The listing builds one solid part. Answer for the finished solid, in the listing's coordinates (mm). Give positions to 0.01 mm unless a question says otherwise; leave off trailing zeros. Loops run counter-clockwise (first coordinate to the right, second up) from the corner with the lowest first, then second, coordinate; pieces in that order, holes last.
Item 1: Each of these flat-tipped pins is pushed along its axis until it touches: pin 1 Ø4 at (x, z) = (-76.2, 139.7) entering from +Y (3 decimals); pin 2 Ø10.5 at (x, z) = (-76.2, -165.1) entering from -Y. Where does it stop, or does it pass through?
Item 2: Consider line 1 along Z through (x, y) = (-25.4, 0.75) (3 decimals); line 2 along X through (y, z) = (1.9, -241.3); line 3 along Z through (x, y) = (6, 2.9) (3 decimals). Determine where each line is inside the solid, lowest interval first.
Item 3: Section A-A, the plane x = -34.5 is taken. Give the vertices of the cut face in (y, z) (3 decimals).
Item 4: Section B-B, the plane y = 2.3 is taken. Give the number of separate pieces and of enclosed holes in the cut face, and give its area (3 significant figures).
Autodesk Inventor part; units mm, degrees
ref_plane "YZ Plane" through (0, 0, 0) normal (1, 0, 0) x (0, 1, 0)
ref_plane "XZ Plane" through (0, 0, 0) normal (0, 1, 0) x (-1, 0, 0)
ref_plane "XY Plane" through (0, 0, 0) normal (0, 0, 1) x (1, 0, 0)
sketch "Sketch1" plane through (0, 0, 0) normal (0, 1, 0) x (-1, 0, 0)
  line L0 (-88.9, -279.4) -> (88.9, -279.4)
  line L1 (88.9, -279.4) -> (88.9, 279.4)
  line L2 (88.9, 279.4) -> (-88.9, 279.4)
  line L3 (-88.9, 279.4) -> (-88.9, -279.4)
  line L4 (-88.9, -279.4) -> (88.9, 279.4) construction
  line L5 (88.9, -279.4) -> (-88.9, 279.4) construction
  point P0 (0, 0)
  dimension "d0" = 558.8
  dimension "d1" = 177.8
extrude "Plate1" add sketch "Sketch1" along normal blind 3.175
sketch "Sketch2" plane through (0, 3.175, 0) normal (0, 1, 0) x (1, 0, 0)
  circle A0 centre (76.2, 266.7) radius 3.302
  line L0 (-88.9, 279.4) -> (88.9, 279.4)
  line L1 (88.9, 279.4) -> (88.9, -279.4)
  circle A1 centre (-68.6663, -258.1933) radius 3.302
  point P0 (0, 0)
  dimension "d3" = 6.604
  dimension "d4" = 12.7
  dimension "d5" = 12.7
  dimension "d14" = 6.604
extrude "Cut1" cut sketch "Sketch2" against normal blind 3.175 contours A0
pattern_linear "Rectangular Pattern1" count 22 spacing 25.4 along (0, 0, 1) of "Cut1"
pattern_linear "Rectangular Pattern2" count 6 spacing 25.4 along (-1, 0, 0) of "Cut1"
sketch "Sketch3" plane through (0, 3.175, 0) normal (0, 1, 0) x (1, 0, 0)
  circle A0 centre (-76.2, -266.7) radius 3.302
  line L0 (-88.9, -279.4) -> (-88.9, 279.4)
  line L1 (88.9, -279.4) -> (-88.9, -279.4)
  point P0 (0, 0)
  dimension "d15" = 6.604
  dimension "d16" = 12.7
  dimension "d17" = 12.7
extrude "Cut2" cut sketch "Sketch3" against normal blind 3.175
pattern_linear "Rectangular Pattern3" count 22 spacing 25.4 along (0, 0, -1) of "Cut2"
pattern_linear "Rectangular Pattern4" count 6 spacing 25.4 along (1, 0, 0) of "Cut2"
sketch "Sketch4" plane through (0, 3.175, 0) normal (0, 1, 0) x (1, 0, 0)
  line L0 (63.5, -88.9) -> (-63.5, -88.9)
  line L1 (-63.5, -88.9) -> (-63.5, 88.9)
  line L2 (-63.5, 88.9) -> (63.5, 88.9)
  line L3 (63.5, 88.9) -> (63.5, -88.9)
  line L4 (63.5, -88.9) -> (-63.5, 88.9) construction
  line L5 (-63.5, -88.9) -> (63.5, 88.9) construction
  point P0 (0, 0)
  dimension "d27" = 127
  dimension "d28" = 177.8
extrude "Cut3" cut sketch "Sketch4" against normal blind 3.175
sketch "Sketch5" plane through (0, 3.175, 0) normal (0, 1, 0) x (1, 0, 0)
  line L0 (-88.9, 279.4) -> (-88.9, -279.4)
  line L1 (-88.9, -279.4) -> (88.9, -279.4)
  line L2 (88.9, -279.4) -> (88.9, -276.225)
  line L3 (88.9, -276.225) -> (-88.9, -276.225)
  line L4 (-88.9, -276.225) -> (-88.9, -279.4)
  line L5 (88.9, 279.4) -> (-88.9, 279.4)
  line L6 (-88.9, 279.4) -> (88.9, 279.4)
  line L7 (88.9, 279.4) -> (88.9, 276.225)
  line L8 (88.9, 276.225) -> (-88.9, 276.225)
  line L9 (-88.9, 276.225) -> (-88.9, 279.4)
  point P0 (0, 0)
  dimension "d31" = 177.8
  dimension "d32" = 3.175
  dimension "d33" = 177.8
  dimension "d34" = 3.175
extrude "Cut4" cut sketch "Sketch5" against normal blind 3.175
equation "\"d6\" = Thickness"
equation "\"d18\" = Thickness"
equation "\"d29\" = Thickness"
equation "\"d35\" = Thickness"
equation "\"d2\" = Thickness"
equation "\"BendRadius\" = Thickness"
equation "\"BendReliefWidth\" = Thickness"
equation "\"BendReliefDepth\" = 0.5 * Thickness"
equation "\"CornerReliefSize\" = 4 * Thickness"
equation "\"MinimumRemnant\" = 2 * Thickness"
equation "\"TransitionRadius\" = BendRadius"
equation "\"JacobiRadiusSize\" = BendRadius"
equation "\"GapSize\" = Thickness"
properties part number "top plate 3" material "Aluminum 6061"
Worked answers:
1. pin 1: passes through
1. pin 2: stops at y = 0
2. line 1: z = -276.225 to -270.002, -263.398 to -88.9, 88.9 to 263.398, 270.002 to 276.225
2. line 2: x = -88.9 to -79.5, -72.9 to 72.9, 79.5 to 88.9
2. line 3: z = -276.225 to -88.9, 88.9 to 276.225
3. outline: (0, -276.225) - (3.175, -276.225) - (3.175, -88.9) - (0, -88.9) - close; (0, 88.9) - (3.175, 88.9) - (3.175, 276.225) - (0, 276.225) - close
4. separate pieces: 1
4. enclosed holes: 55
4. area: 73,800 mm2
